The model under review builds one solid part; all positions refer to its coordinate system, in mm. A direction names the side the tool comes from. Coordinates: 2 decimals unless noted, no trailing zeros. Order: outer loops, then holes, each group sorted by start corner. A loop starts at its lowest first (then second) coordinate and runs counter-clockwise, first axis right, second up. Notation, with made-up numbers: (-12, -6.5) -> (35, -6.5) arc R12 ccw to (35, 12.5) -> close; hole circle Ø11 at (87.25, 40). An arc over 180 degrees is marked (long way). Use one line per item in the form item = value. Start each with the question number.
(1) Take a section at D-D (y = 40). State the section outline as (x, z) points.
(2) Insertion check: pin 1 Ø8 at (y, z) = (12.5, 6) entering from -X; pin 2 Ø13 at (x, y) = (-250, 0) entering from -Z; pin 3 Ø4 at (y, z) = (137.5, 3.5) entering from +X; pin 4 Ø6 at (x, z) = (-316, 4) entering from -Y. Each pin has a flat end and moves straight along its axis. Give the tip position at first contact, or say it passes through.
(3) Take a section at C-C (x = -308). State the section outline as (y, z) points, then the cut area to 3 significant figures.
(4) Take a section at B-B (y = 125). State the section outline as (x, z) points, then the cut area to 3 significant figures.
(5) Take a section at A-A (z = 12.75). State the section outline as (x, y) points, then the cut area to 3 significant figures.
(6) Wall thickness on line 1 along Y through (x, z) = (-218, 11.9); line 2 along Y through (x, z) = (-187.5, 1.9); line 3 along Y through (x, z) = (-141, 1.5): over which ranges is each line inside the solid? List them lowest first.
(7) For faces 4 (the flat face through (-284, 7, 15)), 5 (the cylindrical face through (-363.81, 162.48, 9.93)), list the 3-axis set-ups (+Z, -Z, +X, -X, +Y, -Y) from which the entire face can be reached by the end or side of a thin tool; tool diameter is ignored.
(8) Mouldability with a two-part tool opening along X and no side actions: class faces 1 (the cylindrical face through (-308.199, 226.508, 2.465)), 2 (the flat face through (-217.8, 242.8, 15)), 3 (the cylindrical face through (-274.083, 5.644, 9.93)) as +X half, -X half, draft (parallel to the pull), parting line (faces both ways), or undercut.
Autodesk Fusion 360 part; units mm, degrees
sketch "Sketch5" plane through (0, 0, 0) normal (0, 0, 1) x (1, 0, 0)
  circle A0 centre (-250, 125) radius 150
  line L0 (-250, 125) -> (-250, 250)
  circle A1 centre (-250, 250) radius 8
  circle A2 centre (-312.5, 233.2532) radius 8
  circle A3 centre (-358.2532, 187.5) radius 8
  circle A4 centre (-375, 125) radius 8
  circle A5 centre (-358.2532, 62.5) radius 8
  circle A6 centre (-312.5, 16.7468) radius 8
  circle A7 centre (-250, 0) radius 8
  circle A8 centre (-187.5, 16.7468) radius 8
  circle A9 centre (-141.7468, 62.5) radius 8
  circle A10 centre (-125, 125) radius 8
  circle A11 centre (-141.7468, 187.5) radius 8
  circle A12 centre (-187.5, 233.2532) radius 8
  dimension "d20" = 300
  dimension "d21" = 16
  dimension "d23" = 360
extrude "Extrude4" add sketch "Sketch5" along normal blind 5 makes body 1
sketch "Sketch6" plane through (0, 0, 5) normal (0, 0, 1) x (-1, 0, 0)
  circle A0 centre (125, -125) radius 8
  circle A1 centre (187.5, -233.2532) radius 8
  circle A2 centre (250, -125) radius 150
  circle A3 centre (250, -250) radius 8
  circle A4 centre (375, -125) radius 8
  circle A5 centre (312.5, -233.2532) radius 8
  circle A6 centre (250, 0) radius 8
  circle A7 centre (141.7468, -62.5) radius 8
  circle A8 centre (358.2532, -187.5) radius 8
  circle A9 centre (141.7468, -187.5) radius 8
  circle A10 centre (312.5, -16.7468) radius 8
  circle A11 centre (358.2532, -62.5) radius 8
  circle A12 centre (187.5, -16.7468) radius 8
  arc A13 (187.5, -233.2532) -> (250, -250) centre (260.797, -84.705) ccw
  circle A14 centre (217.9243, -244.708) radius 8
  circle A15 centre (369.708, -157.0757) radius 8
  circle A16 centre (282.0757, -5.292) radius 8
  circle A17 centre (130.292, -92.9243) radius 8
  dimension "d26" = 16
  dimension "d28" = 360
extrude "Extrude5" add sketch "Sketch6" along normal blind 10 contours A13 A14 | A13 A14 | A15 | A16 | A17 bodies 1
sketch "Sketch7" plane through (0, 0, 15) normal (0, 0, 1) x (-1, 0, 0)
  circle A0 centre (282.0757, -5.292) radius 8
  circle A1 centre (282.0757, -5.292) radius 2
  dimension "d31" = 4
sketch "Sketch8" plane through (0, 0, 0) normal (0, 0, 1) x (1, 0, 0)
sketch "Sketch9" plane through (0, 0, 15) normal (0, 0, 1) x (-1, 0, 0)
  circle A0 centre (130.292, -92.9243) radius 8
  circle A1 centre (130.292, -92.9243) radius 2
  dimension "d32" = 4
sketch "Sketch10" plane through (0, 0, 15) normal (0, 0, 1) x (-1, 0, 0)
  circle A0 centre (217.9243, -244.708) radius 8
  circle A1 centre (218, -245) radius 2
  dimension "d33" = 4
sketch "Sketch11" plane through (0, 0, 15) normal (0, 0, 1) x (-1, 0, 0)
  circle A0 centre (369.708, -157.0757) radius 8
  circle A1 centre (369.708, -157.0757) radius 2
  dimension "d34" = 4
extrude "Extrude6" cut sketch "Sketch11" sketch "Sketch10" sketch "Sketch9" sketch "Sketch7" against normal blind 5 contours A1 of sketch 2 contours A1 of sketch 3 contours A1 of sketch 4 contours A1 bodies 1
thread "Thread2" thread offset 0 thread length 10
copy_body "Body->Comp1" bodies 1 removing the originals makes body 2 in component "Component"
sketch "Sketch1" plane through (0, 0, 0) normal (0, 0, 1) x (1, 0, 0)
sketch "Sketch2" plane through (0, 0, 0) normal (1, 0, 0) x (0, 1, 0)
  circle A0 centre (-250, 250) radius 150
  line L0 (-250, 250) -> (-250, 375)
  circle A1 centre (-250, 375) radius 8
  circle A2 centre (-312.5, 358.2532) radius 8
  circle A3 centre (-358.2532, 312.5) radius 8
  circle A4 centre (-375, 250) radius 8
  circle A5 centre (-358.2532, 187.5) radius 8
  circle A6 centre (-312.5, 141.7468) radius 8
  circle A7 centre (-250, 125) radius 8
  circle A8 centre (-187.5, 141.7468) radius 8
  circle A9 centre (-141.7468, 187.5) radius 8
  circle A10 centre (-125, 250) radius 8
  circle A11 centre (-141.7468, 312.5) radius 8
  circle A12 centre (-187.5, 358.2532) radius 8
  line L1 (-250, 375) -> (-187.5, 358.2532)
  line L2 (-250, 375) -> (-218.75, 366.6266)
  circle A13 centre (-220.2756, 367.0354) radius 8
  dimension "d1" = 300
  dimension "d2" = 16
  dimension "d4" = 360
  dimension "d5" = 16
extrude "Extrude1" [suppressed]
sketch "Sketch3" plane through (5, 0, 0) normal (1, 0, 0) x (0, 1, 0)
  circle A0 centre (-141.7468, 187.5) radius 8
  circle A1 centre (-250, 125) radius 8
  circle A2 centre (-250, 250) radius 150
  circle A3 centre (-187.5, 358.2532) radius 8
  circle A4 centre (-250, 375) radius 8
  circle A5 centre (-358.2532, 312.5) radius 8
  circle A6 centre (-312.5, 358.2532) radius 8
  circle A7 centre (-375, 250) radius 8
  circle A8 centre (-358.2532, 187.5) radius 8
  circle A9 centre (-187.5, 141.7468) radius 8
  circle A10 centre (-312.5, 141.7468) radius 8
  circle A11 centre (-141.7468, 312.5) radius 8
  circle A12 centre (-125, 250) radius 8
  line L0 (-250, 375) -> (-187.5, 358.2532)
  circle A13 centre (-218.75, 366.6266) radius 8
  circle A14 centre (-366.6266, 281.25) radius 8
  circle A15 centre (-281.25, 133.3734) radius 8
  circle A16 centre (-133.3734, 218.75) radius 8
  dimension "d8" = 16
  dimension "d10" = 360
extrude "Extrude2" [suppressed]
sketch "Sketch4" plane through (15, 0, 0) normal (1, 0, 0) x (0, 1, 0)
  circle A0 centre (-281.25, 133.3734) radius 8
  circle A1 centre (-281.25, 133.3734) radius 2
  circle A2 centre (-367, 281) radius 2
  circle A3 centre (-218.6865, 366.4726) radius 2
  circle A4 centre (-133.5814, 218.3266) radius 2
  dimension "d13" = 4
  dimension "d14" = 4
  dimension "d15" = 4
extrude "Extrude3" [suppressed]
thread "Thread1" [suppressed]
component "Component" placed x (1, 0, 0) y (0, 1, 0) z (0, 0, 1) at (0, 0, 0)
Findings:
q1.outline = (-373.59, 0) -> (-126.41, 0) -> (-126.41, 5) -> (-373.59, 5) -> close
q2.pin_1 = -353.44
q2.pin_2 = through
q2.pin_3 = -100.37
q2.pin_4 = -11.13
q3.outline = (-13.33, 0) -> (10.13, 0) -> (10.13, 5) -> (-13.33, 5) -> close; (23.36, 0) -> (226.64, 0) -> (226.64, 5) -> (23.36, 5) -> close; (239.87, 0) -> (263.33, 0) -> (263.33, 5) -> (239.87, 5) -> close
q3.area = 1,250 mm²
q4.outline = (-400, 0) -> (-383, 0) -> (-383, 5) -> (-400, 5) -> close; (-367, 0) -> (-133, 0) -> (-133, 5) -> (-367, 5) -> close; (-117, 0) -> (-100, 0) -> (-100, 5) -> (-117, 5) -> close
q4.area = 1,340 mm²
q5.outline = circle Ø16 at (-369.71, 157.08); circle Ø16 at (-282.08, 5.29); circle Ø16 at (-217.92, 244.71); circle Ø16 at (-130.29, 92.92); hole circle Ø4 at (-369.71, 157.08); hole circle Ø4 at (-282.08, 5.29); hole circle Ø4 at (-218, 245); hole circle Ø4 at (-130.29, 92.92)
q5.area = 754 mm²
q6.line_1 = 236.71 to 243, 247 to 252.71
q6.line_2 = -11.36 to 8.75, 24.75 to 225.25, 241.25 to 261.36
q6.line_3 = 21.95 to 54.53, 70.47 to 179.53, 195.47 to 228.05
q7.face_4 = +Z, +X, -X, +Y, -Y
q7.face_5 = +Z
q8.face_1 = undercut
q8.face_2 = draft
q8.face_3 = parting line
